Source: CAD feature listing. Evaluate the final solid. Frame: model axes, mm. Face numbers are marked on the shaded views. A direction names the side the tool comes from. Coordinates: 2 decimals unless noted, no trailing zeros. Loops run counter-clockwise (first coordinate to the right, second up) from the corner with the lowest first, then second, coordinate; pieces in that order, holes last. Notation, with made-up numbers: (7, -27.75) -> (14, -27.75) arc R25 ccw to (14, -1.75) -> close; hole circle Ø11 at (64.25, 35.5). An arc over 180 degrees is marked (long way). Answer as CSV lines item,"result".
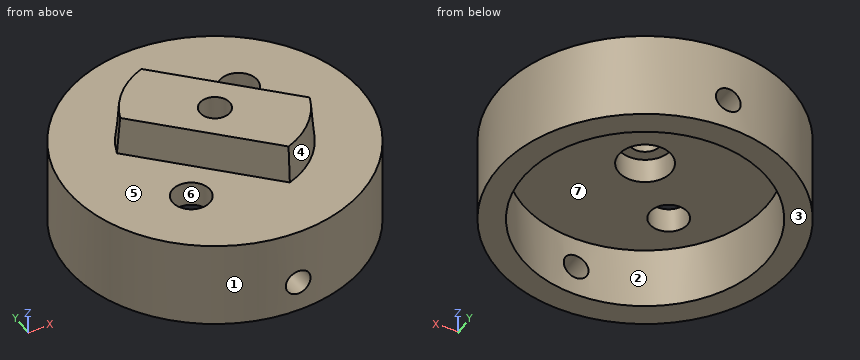
Autodesk Inventor part; units mm, degrees
ref_plane "YZ Plane" through (0, 0, 0) normal (1, 0, 0) x (0, 1, 0)
ref_plane "XZ Plane" through (0, 0, 0) normal (0, 1, 0) x (-1, 0, 0)
ref_plane "XY Plane" through (0, 0, 0) normal (0, 0, 1) x (1, 0, 0)
sketch "Skizze1" plane through (0, 0, 0) normal (0, 0, 1) x (1, 0, 0)
  circle A0 centre (0, 0) radius 9.75
  line L0 (0, 16.45) -> (0, -16.45) construction
  line L1 (-16.45, 0) -> (16.45, 0) construction
  circle A1 centre (4.490128, 4.490128) radius 1.5
  circle A2 centre (0, 0) radius 6.35 construction
  circle A3 centre (-4.490128, -4.490128) radius 1.5
  circle A4 centre (0, 0) radius 11.75
  line L2 (4.490128, 4.490128) -> (0, 0) construction
  circle A5 centre (0, 0) radius 2.1
  circle A6 centre (0, 0) radius 1.2
  arc A7 (2.245874, -6.629936) -> (6.629936, -2.245874) centre (0, 0) ccw
  line L3 (6.629936, -2.245874) -> (-2.245874, 6.629936)
  line L4 (-6.629936, 2.245874) -> (2.245874, -6.629936)
  arc A8 (-2.245874, 6.629936) -> (-6.629936, 2.245874) centre (0, 0) ccw
  arc A9 (-2.245874, 6.629936) -> (-6.629936, 2.245874) centre (0, 0) ccw
  line L5 (0, 0) -> (4.949747, -4.949747) construction
  point P0 (0, -7)
  dimension "d3" = 6.35
  dimension "d0" = 19.5
  dimension "d1" = 3
  dimension "d6" = 360
  dimension "d8" = 2
  dimension "d17" = 45
  dimension "d21" = 4.2
  dimension "d24" = 2.4
  dimension "d76" = 7
  dimension "d122" = 6.2
extrude "Extrusion1" add sketch "Skizze1" against normal blind 7 contours A4
extrude "Extrusion2" add sketch "Skizze1" against normal blind 2 contours A0 | A4 | A5 | A6 | L4 A8 L3 A7
sketch "Skizze2" plane through (0, 0, 0) normal (0, 1, 0) x (-1, 0, 0)
  circle A0 centre (0, -4.5) radius 1
  line L0 (-9.75, 0) -> (9.75, 0)
  point P0 (0, 0)
  dimension "d13" = 2
  dimension "d14" = 4.5
extrude "Extrusion3" cut sketch "Skizze2" along normal through all both and the other way through all
sketch "Skizze1 outline for Extrusion4" plane through (0, 0, 0) normal (0, 0, 1) x (1, 0, 0)
  arc A0 (2.245874, -6.629936) -> (6.629936, -2.245874) centre (0, 0) ccw
  line L0 (-6.629936, 2.245874) -> (2.245874, -6.629936)
  arc A1 (-2.245874, 6.629936) -> (-6.629936, 2.245874) centre (0, 0) ccw
  line L1 (6.629936, -2.245874) -> (-2.245874, 6.629936)
extrude "Extrusion4" add sketch "Skizze1 outline for Extrusion4" along normal blind 3 draft -5
extrude "Extrusion6" cut sketch "Skizze1" along normal through all both and the other way through all contours A6
extrude "Extrusion7" cut sketch "Skizze1" along normal blind 2 from surface at -2 contours A5
properties part number "InputMountingHub"
(1) Cut plane D-D (z = -4.5). Return the cut outline in (x, y).
Computed values:
outline,"(-1, -11.71) -> (-1, -9.7) arc R9.75 cw to (-1, 9.7) -> (-1, 11.71) arc R11.75 ccw to start; (1, -11.71) arc R11.75 ccw to (1, 11.71) -> (1, 9.7) arc R9.75 cw to (1, -9.7) -> close"
(2) Draft query along X for the marked faces 1, 2, 3 and 4. Return one class per face: released by +X, released by -X, zero draft, split by the parting line, or undercut.
Computed values:
face 1,"split by the parting line"
face 2,"undercut"
face 3,"zero draft"
face 4,"released by +X"
(3) Cut plane B-B (x = 0). Return the cut outline in (y, z), then the cut area to 3 significant figures.
Computed values:
outline,"(-11.75, -7) -> (-9.75, -7) -> (-9.75, -5.5) -> (-11.75, -5.5) -> close; (-11.75, -3.5) -> (-9.75, -3.5) -> (-9.75, -2) -> (-2.1, -2) -> (-2.1, 0) -> (-1.2, 0) -> (-1.2, 3) -> (-4.01, 3) -> (-4.38, 0) -> (-11.75, 0) -> close; (1.2, 0) -> (2.1, 0) -> (2.1, -2) -> (9.75, -2) -> (9.75, -3.5) -> (11.75, -3.5) -> (11.75, 0) -> (4.38, 0) -> (4.01, 3) -> (1.2, 3) -> close; (9.75, -7) -> (11.75, -7) -> (11.75, -5.5) -> (9.75, -5.5) -> close"
area,"68.6 mm^2"
(4) Access query for the marked faces 5, 6 and 7. Directions: +Z, -Z, +X, -X, +Y, -Y. A direction counts if a zero-diameter tool reaches every point of the face in a straight line with its end or side. Return the directions, or none.
Computed values:
face 5,"+Z"
face 6,"+Z, -Z"
face 7,"-Z"
(5) Cut plane A-A (y = 0). Return the cut outline in (x, z), then the cut area to 3 significant figures.
Computed values:
outline,"(-11.75, -7) -> (-9.75, -7) -> (-9.75, -2) -> (-2.1, -2) -> (-2.1, 0) -> (-1.2, 0) -> (-1.2, 3) -> (-4.01, 3) -> (-4.38, 0) -> (-11.75, 0) -> close; (1.2, 0) -> (2.1, 0) -> (2.1, -2) -> (9.75, -2) -> (9.75, -7) -> (11.75, -7) -> (11.75, 0) -> (4.38, 0) -> (4.01, 3) -> (1.2, 3) -> close"
area,"76.6 mm^2"
(6) Material intervals for L1, parallel to X at y = 0.25, z = -4.25; L2, parallel to Y at x = 0, z = -0.55; L3, parallel to Z at x = 7.25, y = 7.5, sorted ascending. Write a range as [from, to].
Computed values:
L1,"[-11.75, -9.75], [9.75, 11.75]"
L2,"[-11.75, -2.1], [2.1, 11.75]"
L3,"[-7, 0]"
(7) Cut plane C-C (z = -6). Return the cut outline in (x, y), then the cut area to 3 significant figures.
Computed values:
outline,"circle Ø23.5 at (0, 0); hole circle Ø19.5 at (0, 0)"
area,"135 mm^2"
(8) Pin query (flat end, axial travel): pin 1 Ø1.5 at (x, y) = (6.5, 8.5) entering from +Z; pin 2 Ø1.8 at (x, z) = (0, -4.5) entering from -Y; pin 3 Ø2.5 at (x, z) = (0, -4.5) entering from -Y; pin 4 Ø4 at (y, z) = (-6, -5.5) entering from +X. Return the tip coordinate at first contact, or that it passes through.
Computed values:
pin 1,"z = 0"
pin 2,"through"
pin 3,"y = -11.75"
pin 4,"x = 11.05"
